from build123d import *

# Parameters (mm, degrees)
F1_DEPTH = 20
F2_R     = 5
F2_R_2   = 2
F3_DEPTH = 25
F4_DEPTH = 25


with BuildPart() as f1:
    # F0 (on Top) → F1 (new body)
    with BuildSketch(Plane.XY):
        with BuildLine():
            Line((-9.9256848916, -12.5), (-7.5, -12.5))
            Line((-7.5, -12.5), (7.5, -12.5))
            Line((7.5, -12.5), (9.9256848916, -12.5))
            add(Edge.make_bspline(
                [(7.5, -6.2737814151), (8.087411693, -8.3720675571), (8.674823386, -10.4703536991), (9.9256848916, -12.5)],
                knots=[0, 0, 0, 0, 0.4559339128, 0.4559339128, 0.4559339128, 0.4559339128], degree=3))
            Line((7.5, -6.2737814151), (7.5, 12.5))
            Line((7.5, 12.5), (-7.5, 12.5))
            Line((-7.5, 12.5), (-7.5, -6.2737814151))
            add(Edge.make_bspline(
                [(-7.5, -6.2737814151), (-8.087411693, -8.3720675571), (-8.674823386, -10.4703536991), (-9.9256848916, -12.5)],
                knots=[0, 0, 0, 0, 0.4559339128, 0.4559339128, 0.4559339128, 0.4559339128], degree=3))
        make_face()
    extrude(amount=F1_DEPTH)

    # F2 (on Front) → F3 (cut)
    with BuildSketch(Plane.XZ):
        with Locations((0, 10)):
            Circle(F2_R)
        with Locations((0, 10)):
            Circle(F2_R_2, mode=Mode.SUBTRACT)
        with Locations((0, 10)):
            Circle(F2_R_2)
    extrude(amount=F3_DEPTH, mode=Mode.SUBTRACT)

    # F2 (on Front) → F4 (cut)
    with BuildSketch(Plane.XZ):
        with Locations((0, 10)):
            Circle(F2_R_2)
    extrude(amount=-F4_DEPTH, mode=Mode.SUBTRACT)


solid = f1.part
Part model, mm, in its own coordinate system. A direction names the side the tool comes from. Coordinates: 2 decimals unless noted, no trailing zeros. Order: outer loops, then holes, each group sorted by start corner. A loop starts at its lowest first (then second) coordinate and runs counter-clockwise, first axis right, second up. Notation, with made-up numbers: M 79,39 L 137,39 A20 ccw 137,72 Z; hole C 80.25,-26.75 d10. An arc over 180 degrees is marked long. Use a Markdown table: item, result.
(1) Pull direction Z, two halves, no side cores. Call faces 1 (the flat face through (0, 0, 20)), 2 (the flat face through (-7.5, 3, 10)), 3 (the cylindrical face through (0, 6, 12)), 4 (the flat face through (0, 0, 0)): released by +Z, released by -Z, zero draft, split by the parting line, or undercut.
A:
| item | result |
|---|---|
| face 1 | released by +Z |
| face 2 | zero draft |
| face 3 | undercut |
| face 4 | released by -Z |
(2) Tool access for faces 5 (the cylindrical face through (-0.651, -6.162, 14.957)), 6 (the flat face through (7.5, 3, 10)), 7 (the flat face through (-5, -12.5, 8)): list every direction of +Z, -Z, +X, -X, +Y, -Y with a clear straight run to the whole face (end or side of a thin tool).
A:
| item | result |
|---|---|
| face 5 | -Y |
| face 6 | +Z, -Z, +X, +Y |
| face 7 | +Z, -Z, +X, -X, -Y |
(3) Probe L1, parallel to X at y = -5, z = 10; L2, parallel to Z at x = 0, y = -2.25; L3, parallel to Z at x = 0, y = 9.75. List the from-to ranges inside material, lowest first.
A:
| item | result |
|---|---|
| L1 | x = -7.5 to -5, 5 to 7.5 |
| L2 | z = 0 to 5, 15 to 20 |
| L3 | z = 0 to 8, 12 to 20 |
(4) Cut at D-D on x = -2.75. Write the cut outline in (y, z), then the cut area to 3 significant figures.
A:
| item | result |
|---|---|
| outline | M -12.5,0 L 12.5,0 L 12.5,20 L -12.5,20 L -12.5,14.18 L 0,14.18 L 0,5.82 L -12.5,5.82 Z |
| area | 396 mm^2 |
(5) Cut at B-B on y = -1.5. Write the cut outline in (x, z), then the cut area to 3 significant figures.
A:
| item | result |
|---|---|
| outline | M -7.5,0 L 7.5,0 L 7.5,20 L -7.5,20 Z; hole C 0,10 d10 |
| area | 221 mm^2 |
(6) Cut at A-A on x = 0. Write the cut outline in (y, z).
A:
| item | result |
|---|---|
| outline | M -12.5,0 L 12.5,0 L 12.5,8 L 0,8 L 0,5 L -12.5,5 Z; M -12.5,15 L 0,15 L 0,12 L 12.5,12 L 12.5,20 L -12.5,20 Z |
(7) Cut at C-C on y = 3.5. Write the cut outline in (x, z).
A:
| item | result |
|---|---|
| outline | M -7.5,0 L 7.5,0 L 7.5,20 L -7.5,20 Z; hole C 0,10 d4 |
(8) Flat gauge pins, fed straight in: pin 1 (9.5 mm diameter, centred on y = 6, z = 9, fed in from +X); pin 2 (2 mm diameter, centred on y = -5, z = 12.5, fed in from -X); pin 3 (6.5 mm diameter, centred on x = 0, z = 10, fed in from -Y). Where does each tip first touch, or does it go through?
A:
| item | result |
|---|---|
| pin 1 | stops at x = 7.5 |
| pin 2 | stops at x = -7.5 |
| pin 3 | stops at y = 0 |
